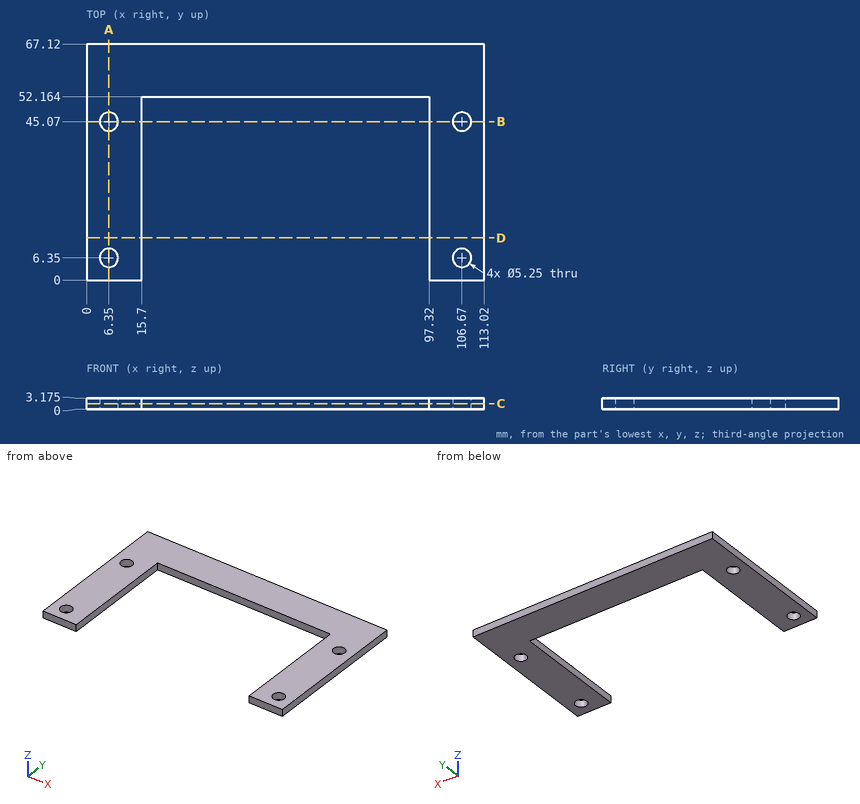
Can you work these out from the drawing? Everything is in mm from the part's minimum corner. Give positions to 0.01 mm unless a question says otherwise; leave off trailing zeros. Loops run counter-clockwise (first coordinate to the right, second up) from the corner with the lowest first, then second, coordinate; pieces in that order, holes last. Notation, with made-up numbers: (19.5, 34) - (30.5, 34) arc R28 ccw to (30.5, 62) - close; hole circle Ø10 at (-20.5, 10). An arc over 180 degrees is marked (long way). Use one line per item in the form item = value.
1. I want a section at D-D (y = 12). Please give me the cut outline in (x, z) (1 decimal).
Response values:
outline = (0, 0) - (15.7, 0) - (15.7, 3.2) - (0, 3.2) - close; (97.3, 0) - (113, 0) - (113, 3.2) - (97.3, 3.2) - close
2. I need wall thicknesses on probe 1 along Y at (x, z) = (6.35, 2.45) (1 decimal); probe 2 along X at (y, z) = (18, 1.65); probe 3 along Y at (x, z) = (73.5, 2.3). Which ranges of each line are inside material? Lowest first, please.
Response values:
probe_1 = 0 to 3.7, 9 to 42.4, 47.7 to 67.1
probe_2 = 0 to 15.7, 97.32 to 113.02
probe_3 = 52.16 to 67.12
3. I want a section at A-A (x = 6.35). Please give me the cut outline in (y, z) (1 decimal).
Response values:
outline = (0, 0) - (3.7, 0) - (3.7, 3.2) - (0, 3.2) - close; (9, 0) - (42.4, 0) - (42.4, 3.2) - (9, 3.2) - close; (47.7, 0) - (67.1, 0) - (67.1, 3.2) - (47.7, 3.2) - close
4. I want a section at B-B (y = 45.07). Please give me the cut outline in (x, z) (1 decimal).
Response values:
outline = (0, 0) - (3.7, 0) - (3.7, 3.2) - (0, 3.2) - close; (9, 0) - (15.7, 0) - (15.7, 3.2) - (9, 3.2) - close; (97.3, 0) - (104, 0) - (104, 3.2) - (97.3, 3.2) - close; (109.3, 0) - (113, 0) - (113, 3.2) - (109.3, 3.2) - close
5. I want a section at C-C (z = 1.65). Give the number of separate pieces and of enclosed holes in the cut face, and give its area (3 significant figures).
Response values:
separate_pieces = 1
enclosed_holes = 4
area = 3,240 mm²
6. I'm going to push a flat-ended pin straight in: pin 1 Ø1 at (x, z) = (73.5, 2) entering from -Y. Where does the tip first touch, or does it pass through?
Response values:
pin_1 = 52.16
